from build123d import *

# Parameters (mm, degrees)
BOSS_EXTRUDE1_DEPTH = 12.7
SKETCH2_R           = 6.35
CUT_EXTRUDE1_DEPTH  = 182.323455578
CUT_EXTRUDE10_DEPTH = 182.323455578


with BuildPart() as part:
    # Sketch1 → Boss-Extrude1 (new body)
    with BuildSketch(Plane(origin=(0, 0, 0), x_dir=(1, 0, 0), z_dir=(0, 1, 0))):
        with BuildLine():
            Line((-131.471489953, 109.23134636), (71.728510047, 109.23134636))
            ThreePointArc((71.728510047, 109.23134636), (80.708766168, 105.511602481), (84.428510047, 96.53134636))
            Line((84.428510047, 96.53134636), (84.428510047, 38.349564826))
            ThreePointArc((84.428510047, 38.349564826), (83.442873319, 33.444088994), (80.638952072, 29.300033185))
            Line((80.638952072, 29.300033185), (10.746499625, -39.518185281))
            ThreePointArc((10.746499625, -39.518185281), (6.650668081, -42.220654573), (1.836057601, -43.16865364))
            Line((1.836057601, -43.16865364), (-63.841823784, -43.16865364))
            ThreePointArc((-63.841823784, -43.16865364), (-68.748013198, -42.182718068), (-72.892440933, -39.377993078))
            Line((-72.892440933, -39.377993078), (-140.522107103, 29.324094297))
            ThreePointArc((-140.522107103, 29.324094297), (-143.22378415, 33.419539146), (-144.171489953, 38.233433734))
            Line((-144.171489953, 38.233433734), (-144.171489953, 96.53134636))
            ThreePointArc((-144.171489953, 96.53134636), (-140.451746074, 105.511602481), (-131.471489953, 109.23134636))
        make_face()
    extrude(amount=BOSS_EXTRUDE1_DEPTH)

    # Sketch2 → Cut-Extrude1 (cut, through all)
    with BuildSketch(Plane(origin=(0, 12.7, 0), x_dir=(1, 0, 0), z_dir=(0, 1, 0))):
        with Locations(Location((-69.102883091, -30.46865364, 0), (0, 0, 270))):
            Circle(SKETCH2_R)
        with Locations(Location((7.097116909, -30.46865364, 0), (0, 0, 270))):
            Circle(SKETCH2_R)
        with Locations(Location((-67.971489953, 96.53134636, 0), (0, 0, 270))):
            Circle(SKETCH2_R)
        with Locations(Location((8.228510047, 96.53134636, 0), (0, 0, 270))):
            Circle(SKETCH2_R)
        with Locations(Location((-67.971489286, 33.021266411, 0), (0, 0, 270))):
            Circle(SKETCH2_R)
        with Locations(Location((8.228510047, 33.03134636, 0), (0, 0, 270))):
            Circle(SKETCH2_R)
        with Locations(Location((-131.471489953, 96.53134636, 0), (0, 0, 270))):
            Circle(SKETCH2_R)
        with Locations(Location((-131.471489953, 33.03134636, 0), (0, 0, 270))):
            Circle(SKETCH2_R)
        with Locations(Location((71.728510047, 96.53134636, 0), (0, 0, 270))):
            Circle(SKETCH2_R)
        with Locations(Location((71.728510047, 33.03134636, 0), (0, 0, 270))):
            Circle(SKETCH2_R)
        with Locations(Location((-29.871490619, 33.03134636, 0), (0, 0, 270))):
            Circle(SKETCH2_R)
    extrude(amount=-CUT_EXTRUDE1_DEPTH, mode=Mode.SUBTRACT)

    # Sketch3 → Cut-Extrude10 (cut, through all)
    with BuildSketch(Plane(origin=(0, 12.7, 0), x_dir=(1, 0, 0), z_dir=(0, 1, 0))):
        Polygon((-132.534139195, 32.962602464), (-69.102883091, -30.46865364), (7.097116909, -30.46865364), (71.522699324, 33.956928775), align=None)
    extrude(amount=-CUT_EXTRUDE10_DEPTH, mode=Mode.SUBTRACT)


solid = part.part
Could you check a few things on this model? Use its own coordinates, in mm. A direction names the side the tool comes from. Give positions to 0.01 mm unless a question says otherwise; leave off trailing zeros. Write each loop counter-clockwise with the first axis right and the second up, starting at its lowest first coordinate (ties: lowest second). Pieces come first, ordered by that corner, then holes. Notation, with made-up numbers: (40.25, 34.25) -> (44.25, 34.25) arc R10 cw to (44.25, 49.25) -> close; hole circle Ø7 at (33, -18.5). An arc over 180 degrees is marked (long way). Answer as a JSON object with one key per item and string values.
Q1. Suppose I cut it at C-C on x = 69.5. Write out the boundary of the cut face in (y, z), then the cut area to 3 significant figures.
Taken from the geometry:
{"outline": "(0, -109.23) -> (12.7, -109.23) -> (12.7, -102.48) -> (0, -102.48) -> close; (0, -90.59) -> (12.7, -90.59) -> (12.7, -38.98) -> (0, -38.98) -> close; (0, -27.09) -> (12.7, -27.09) -> (12.7, -18.33) -> (0, -18.33) -> close", "area": "852 mm²"}
Q2. Please list where these lines run through material, in increasing order: L1, parallel to X at y = 1.25, z = -35.5; L2, parallel to Z at x = -1, y = 4.5; L3, parallel to Z at x = -126, y = 9.5.
Taken from the geometry:
{"L1": "x = -143.87 to -137.32, -125.62 to -73.82, -62.13 to -35.72, -24.02 to 2.38, 14.08 to 65.88, 77.58 to 84.1", "L2": "z = -109.23 to -33.6, 30.47 to 43.17", "L3": "z = -109.23 to -99.75, -93.31 to -36.25, -26.43 to -14.57"}
Q3. Will these pins go through, and if not, where does the flat tip stop? pin 1 Ø11.5 at (x, z) = (71.73, -33.03) entering from -Y; pin 2 Ø3 at (x, y) = (-86, 9) entering from +Z; pin 3 Ø4 at (x, y) = (-113.5, 7) entering from +Z.
Taken from the geometry:
{"pin 1": "passes through", "pin 2": "stops at z = 27.59", "pin 3": "stops at z = 0.16"}
Q4. Suppose I cut it at A-A on x = -43. Write out the boundary of the cut face in (y, z).
Taken from the geometry:
{"outline": "(0, -109.23) -> (12.7, -109.23) -> (12.7, -33.4) -> (0, -33.4) -> close; (0, 30.47) -> (12.7, 30.47) -> (12.7, 43.17) -> (0, 43.17) -> close"}
Q5. Suppose I cut it at D-D on y = 8.5. Count the separate pieces of the cut face and the enclosed holes in it, then the cut area to 3 significant figures.
Taken from the geometry:
{"separate pieces": "1", "enclosed holes": "5", "area": "18,900 mm²"}
Q6. Which directions (+Z, -Z, +X, -X, +Y, -Y) give clear straight access to the entire face, cutting with the end or side of a thin tool? Please do faces 1 (the cylindrical face through (-29.77, 6.44, -39.38)), 2 (the flat face through (-31, 6, -109.231)).
Taken from the geometry:
{"face 1": "+Y, -Y", "face 2": "-Z, +X, -X, +Y, -Y"}
Q7. Suppose I cut it at B-B on z = -22. Write out the boundary of the cut face in (x, y), then the cut area to 3 significant figures.
Taken from the geometry:
{"outline": "(-133.31, 0) -> (-121.57, 0) -> (-121.57, 12.7) -> (-133.31, 12.7) -> close; (59.57, 0) -> (73.22, 0) -> (73.22, 12.7) -> (59.57, 12.7) -> close", "area": "323 mm²"}
Q8. We'd pull the mould along X, two halves only. Please class faces 3 (the cylindrical face through (10.136, 6.439, -90.475)), 4 (the flat face through (-144.171, 6, -67)), 5 (the flat face through (-28, 12.7, -51)): released by +X, released by -X, zero draft, split by the parting line, or undercut.
Taken from the geometry:
{"face 3": "undercut", "face 4": "released by -X", "face 5": "zero draft"}
